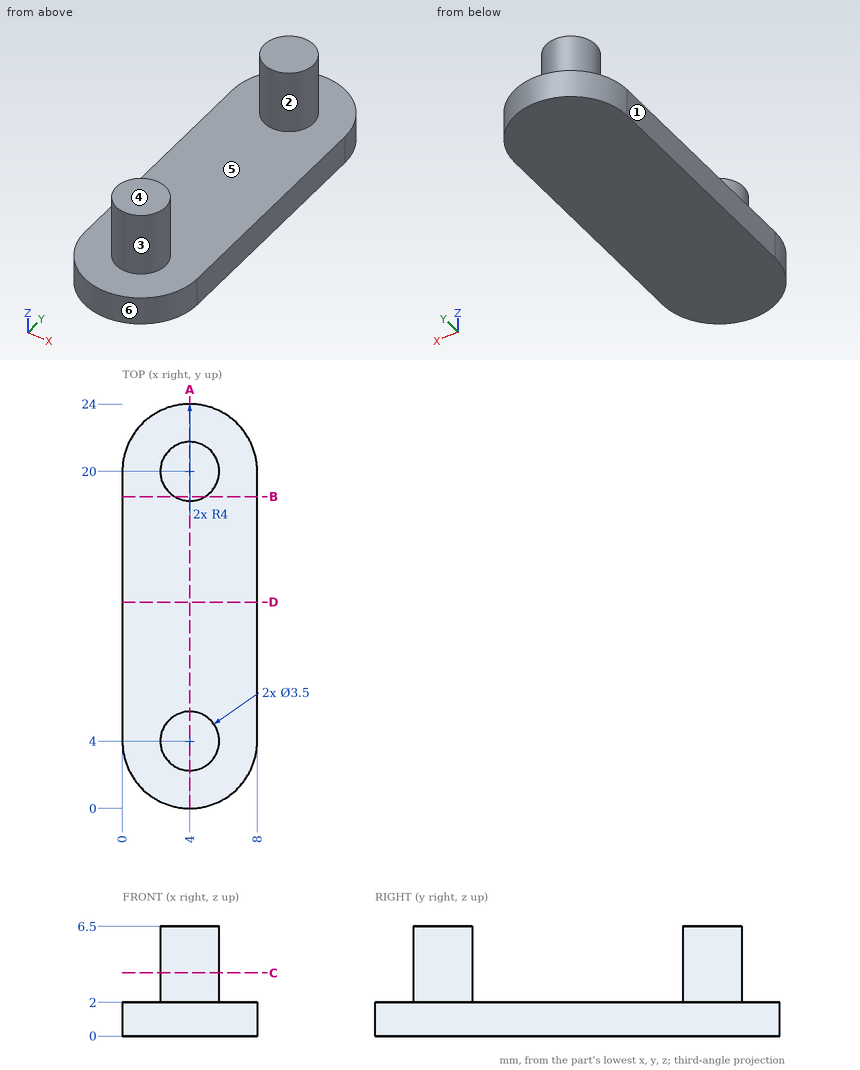
Part print with two shaded views. Sizes in mm from the minimum x, y, z corner. A direction names the side the tool comes from. Coordinates: 2 decimals unless noted, no trailing zeros. Loops run counter-clockwise (first coordinate to the right, second up) from the corner with the lowest first, then second, coordinate; pieces in that order, holes last. Notation, with made-up numbers: (66, 0) -> (72, 0) arc R11 cw to (72, 16) -> close; hole circle Ø5 at (-1.75, 46.5). An arc over 180 degrees is marked (long way). Answer as a JSON object with one key per item and string values.
Q1. Cut at D-D (y = 12.25). List the corners of the cut face in (x, z).
Report:
{"outline": "(0, 0) -> (8, 0) -> (8, 2) -> (0, 2) -> close"}
Q2. Cut at C-C (z = 3.75). List the corners of the cut face in (x, y).
Report:
{"outline": "circle Ø3.5 at (4, 4); circle Ø3.5 at (4, 20)"}
Q3. Pull direction Y, two halves, no side cores. Call the marked faces 3, 4, 5 and 6: released by +Y, released by -Y, zero draft, split by the parting line, or undercut.
Report:
{"face 3": "undercut", "face 4": "zero draft", "face 5": "undercut", "face 6": "released by -Y"}
Q4. Cut at B-B (y = 18.5). List the corners of the cut face in (x, z), and give its area (3 significant figures).
Report:
{"outline": "(0, 0) -> (8, 0) -> (8, 2) -> (4.9, 2) -> (4.9, 6.5) -> (3.1, 6.5) -> (3.1, 2) -> (0, 2) -> close", "area": "24.1 mm2"}
Q5. Cut at A-A (x = 4). List the corners of the cut face in (y, z), and give its area (3 significant figures).
Report:
{"outline": "(0, 0) -> (24, 0) -> (24, 2) -> (21.75, 2) -> (21.75, 6.5) -> (18.25, 6.5) -> (18.25, 2) -> (5.75, 2) -> (5.75, 6.5) -> (2.25, 6.5) -> (2.25, 2) -> (0, 2) -> close", "area": "79.5 mm2"}
Q6. Probe probe 1 along Z at (x, y) = (5.75, 22); probe 2 along Y at (x, z) = (4.25, 5); probe 3 along Y at (x, z) = (5.5, 4.75). List the from-to ranges inside material, lowest first.
Report:
{"probe 1": "z = 0 to 2", "probe 2": "y = 2.27 to 5.73, 18.27 to 21.73", "probe 3": "y = 3.1 to 4.9, 19.1 to 20.9"}
Q7. 3-axis set-ups, long thin cutter, end or side, ignore diameter. For the marked faces 1 and 2: which of +Z, -Z, +X, -X, +Y, -Y reach the whole face in a straight line?
Report:
{"face 1": "+Z, -Z, -X, +Y, -Y", "face 2": "+Z"}
